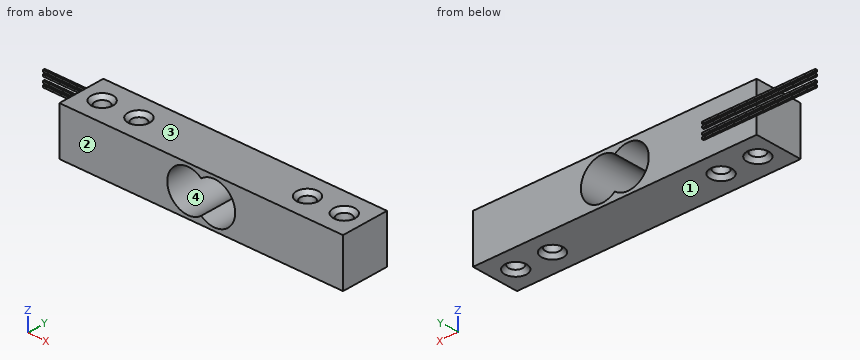
from build123d import *

# Parameters (mm, degrees)
F0_W          = 75.2
F0_H          = 12.7
F1_DEPTH      = 6.35
F1_DEPTH_BACK = 6.35
F3_DEPTH      = 25
F4_W          = 30
F4_H          = 0.5
F5_DEPTH      = 0.5
F6_R          = 1.875
F7_DEPTH      = 25
F8_SIZE       = 1


with BuildPart() as f1:
    # F0 (on Top) → F1 (new body, two sides)
    with BuildSketch(Plane.XY) as f1_sk:
        Rectangle(F0_W, F0_H)
    extrude(amount=F1_DEPTH)
    extrude(f1_sk.sketch, amount=-F1_DEPTH_BACK)

    # F2 (on face) → F3 (cut)
    with BuildSketch(Plane.XZ.offset(6.35)):
        with BuildLine():
            ThreePointArc((0, 4.242641), (-9, 0), (0, -4.242641))
            ThreePointArc((0, -4.242641), (9, 0), (0, 4.242641))
        make_face()
    extrude(amount=-F3_DEPTH, mode=Mode.SUBTRACT)

    # F4 (on face) → F5 (join)
    with BuildSketch(Plane(origin=(0, 6.35, 0), x_dir=(-1, 0, 0), z_dir=(0, 1, 0))):
        with Locations((38.6, 1.75)):
            Rectangle(F4_W, F4_H)
        with Locations((38.6, 0.75)):
            Rectangle(F4_W, F4_H)
        with Locations((38.6, -0.75)):
            Rectangle(F4_W, F4_H)
        with Locations((38.6, -1.75)):
            Rectangle(F4_W, F4_H)
    extrude(amount=F5_DEPTH)

    # F6 (on face) → F7 (cut)
    with BuildSketch(Plane.XY.offset(6.35)):
        with Locations((32.1, 0)):
            Circle(F6_R)
        with Locations((22.35, 0)):
            Circle(F6_R)
        with Locations((-22.35, 0)):
            Circle(F6_R)
        with Locations((-32.1, 0)):
            Circle(F6_R)
    extrude(amount=-F7_DEPTH, mode=Mode.SUBTRACT)

    # F8
    f8_edges = [f1.edges().sort_by_distance(p)[0] for p in [
        (30.225, 0, 6.35),
        (20.475, 0, 6.35),
        (-24.225, 0, 6.35),
        (-33.975, 0, 6.35),
        (-33.975, 0, -6.35),
        (-24.225, 0, -6.35),
        (20.475, 0, -6.35),
        (30.225, 0, -6.35),
    ]]
    chamfer(f8_edges, length=F8_SIZE)


solid = f1.part
Check sheet for the modelled part. Datum: model origin and axes. Units: mm. Face numbers are marked on the shaded views. Give positions to 0.01 mm unless a question says otherwise; leave off trailing zeros. Order: outer loops, then holes, each group sorted by start corner. A loop starts at its lowest first (then second) coordinate and runs counter-clockwise, first axis right, second up. Notation, with made-up numbers: M 28.25,17.5 L 41.25,17.5 A23 cw 41.25,31.5 Z; hole C 24.5,10.5 d6. An arc over 180 degrees is marked long. Answer as CSV lines item,"result". Start each with the question number.
Item 1: Cross-section at C-C on x = -3.5. Enter the section's corners in (y, z), plus the area to 3 significant figures.
Item 2: Cross-section at A-A on x = -32.1. Enter the section's corners in (y, z) (3 decimals).
Item 3: Mould release check, pull along Z, two halves, no side actions. Record for the marked faces 1, 2, 3 and 4: +Z half, -Z half, draft (parallel to the pull), parting line (faces both ways), or undercut.
Item 4: Gauge pin test, flat ends, axial feed: P1, Ø3, axis at x = 16.5, z = -1.5, coming from the +Y side; P2, Ø5, axis at x = -22.35, y = 0, coming from the -Z side (3 decimals); P3, Ø0.6, axis at x = -41.5, y = 6.5, coming from the -Z side. Record the tip position at first contact, or that the pin passes through.
Item 5: Thickness scan on line 1 (X direction, y = -0.25, z = 0); line 2 (Y direction, x = -32.1, z = -1.75) (3 decimals); line 3 (Z direction, x = -3.5, y = -3). Record the ranges inside material, lowest first. Write a range as [from, to].
Item 6: Cross-section at B-B on z = -3. Enter the section's corners in (x, y) (3 decimals).
Item 7: Cross-section at D-D on z = 2.75. Enter the section's corners in (x, y) (3 decimals), plus the area to 3 significant figures.
Established:
1,outline,"M -6.35,-6.35 L 6.35,-6.35 L 6.35,-5.5 L -6.35,-5.5 Z; M -6.35,5.5 L 6.35,5.5 L 6.35,6.35 L -6.35,6.35 Z"
1,area,"21.6 mm^2"
2,outline,"M -6.35,-6.35 L -2.875,-6.35 L -1.875,-5.35 L -1.875,5.35 L -2.875,6.35 L -6.35,6.35 Z; M 1.875,-5.35 L 2.875,-6.35 L 6.35,-6.35 L 6.35,-2 L 6.85,-2 L 6.85,-1.5 L 6.35,-1.5 L 6.35,-1 L 6.85,-1 L 6.85,-0.5 L 6.35,-0.5 L 6.35,0.5 L 6.85,0.5 L 6.85,1 L 6.35,1 L 6.35,1.5 L 6.85,1.5 L 6.85,2 L 6.35,2 L 6.35,6.35 L 2.875,6.35 L 1.875,5.35 Z"
3,face 1,"-Z half"
3,face 2,"draft"
3,face 3,"+Z half"
3,face 4,"undercut"
4,P1,"stops at y = 6.35"
4,P2,"stops at z = -5.975"
4,P3,"stops at z = -2"
5,line 1,"x = [-37.6, -33.96], [-30.24, -24.21], [-20.49, -9], [9, 20.49], [24.21, 30.24], [33.96, 37.6]"
5,line 2,"y = [-6.35, -1.875], [1.875, 6.85]"
5,line 3,"z = [-6.35, -5.5], [5.5, 6.35]"
6,outline,"M -37.6,-6.35 L -8.11,-6.35 L -8.11,6.35 L -37.6,6.35 Z; M 8.11,-6.35 L 37.6,-6.35 L 37.6,6.35 L 8.11,6.35 Z; hole C -32.1,0 d3.75; hole C -22.35,0 d3.75; hole C 22.35,0 d3.75; hole C 32.1,0 d3.75"
7,outline,"M -37.6,-6.35 L -8.263,-6.35 L -8.263,6.35 L -37.6,6.35 Z; M 8.263,-6.35 L 37.6,-6.35 L 37.6,6.35 L 8.263,6.35 Z; hole C -32.1,0 d3.75; hole C -22.35,0 d3.75; hole C 22.35,0 d3.75; hole C 32.1,0 d3.75"
7,area,"701 mm^2"
